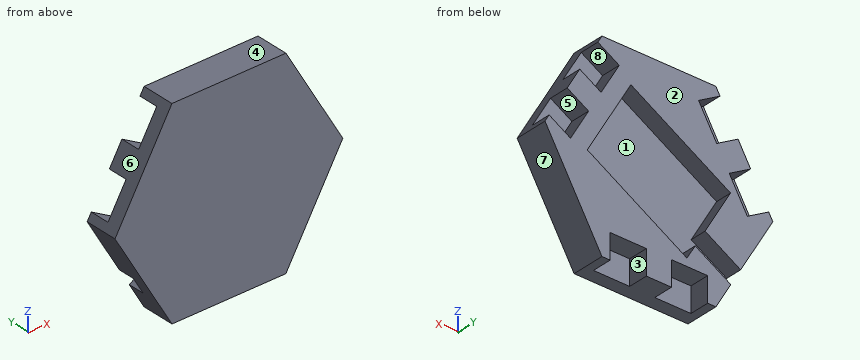
```python
from build123d import *

# Parameters (mm, degrees)
BOSS_EXTRUDE1_DEPTH     = 20
SKETCH2_W               = 22
SKETCH2_H               = 15
CUT_EXTRUDE1_DEPTH      = 12
CUT_EXTRUDE2_DEPTH      = 94.808315196
CUT_EXTRUDE2_DEPTH_BACK = 10


with BuildPart() as part:
    # Sketch1 → Boss-Extrude1 (new body)
    with BuildSketch(Plane(origin=(0, 0, 0), x_dir=(1, 0, 0), z_dir=(0, 1, 0))):
        Polygon((69.282032303, 0), (34.641016151, 60), (-34.641016151, 60), (-69.282032303, 0), (-34.641016151, -60), (34.641016151, -60), align=None)
    extrude(amount=BOSS_EXTRUDE1_DEPTH)

    # Sketch2 → Cut-Extrude1 (cut)
    with BuildSketch(Plane(origin=(0, 20, 0), x_dir=(1, 0, 0), z_dir=(0, 1, 0))):
        with Locations((-18.641016151, 52.5)):
            Rectangle(SKETCH2_W, SKETCH2_H)
        with Locations((18.641016151, 52.5)):
            Rectangle(SKETCH2_W, SKETCH2_H)
        Polygon((66.782032303, -4.330127019), (53.791651246, 3.169872981), (42.791651246, -15.882685902), (55.782032303, -23.382685902), align=None)
        Polygon((48.141016151, -36.617314098), (35.150635095, -29.117314098), (24.150635095, -48.169872981), (37.141016151, -55.669872981), align=None)
        Polygon((-37.141016151, -55.669872981), (-24.150635095, -48.169872981), (-35.150635095, -29.117314098), (-48.141016151, -36.617314098), align=None)
        Polygon((-55.782032303, -23.382685902), (-42.791651246, -15.882685902), (-53.791651246, 3.169872981), (-66.782032303, -4.330127019), align=None)
    extrude(amount=-CUT_EXTRUDE1_DEPTH, mode=Mode.SUBTRACT)

    # Sketch3 → Cut-Extrude2 (cut, two sides: drawn at the far end of the back side and taken through both)
    with BuildSketch(Plane(origin=(0, 20, 0), x_dir=(1, 0, 0), z_dir=(0, 1, 0)).offset(-CUT_EXTRUDE2_DEPTH_BACK)):
        Polygon((-43.560889132, -5.4496732), (17.060889132, -40.4496732), (43.560889132, 5.4496732), (-17.060889132, 40.4496732), align=None)
        Polygon((-22.060889132, 31.789419162), (-28.060889132, 21.397114317), (-49.711524227, 33.897114317), (-43.711524227, 44.289419162), align=None)
    extrude(amount=CUT_EXTRUDE2_DEPTH + CUT_EXTRUDE2_DEPTH_BACK, mode=Mode.SUBTRACT)


solid = part.part
```
CAD build for the part. Positions are in the model's coordinates, mm. Face numbers are marked on the shaded views. A direction names the side the tool comes from. Round coordinates to 2 decimals unless told otherwise and drop trailing zeros. Write each loop counter-clockwise with the first axis right and the second up, starting at its lowest first coordinate (ties: lowest second). Pieces come first, ordered by that corner, then holes. Notation, with made-up numbers: (44, -20.75) - (63, -20.75) arc R7 cw to (63, -15.75) - close; hole circle Ø4 at (-5.75, 27). An arc over 180 degrees is marked (long way). Write item = value, one per line. Start each with the question number.
Q1. Which spindle directions (+Z, -Z, +X, -X, +Y, -Y) get a long thin tool onto all of the face, cutting with end or side? Do the marked faces 1, 2, 3, 4 and 5. Say none if no direction does.
Q2. Band-saw the part on A-A (y = 3.5). Give the cut face in (x, z), then the cut area to 3 significant figures.
Q3. Drop flat-ended pins along their axis: pin 1 (5 mm diameter, centred on x = -4, z = 42.5, fed in from -Y); pin 2 (5 mm diameter, centred on y = 14.5, z = -31.5, fed in from +X); pin 3 (6 mm diameter, centred on y = 15, z = -55, fed in from -X); pin 4 (3.5 mm diameter, centred on y = 14.5, z = -52.5, fed in from -X). Give the stop position or say it passes through.
Q4. Band-saw the part on C-C (z = -50). Give the cut face in (x, y).
Q5. Band-saw the part on D-D (z = 43). Give the cut face in (x, y).
Q6. Probe L1, parallel to X at y = 11, z = -33; L2, parallel to Z at x = -36.5, y = 13; L3, parallel to Y at x = -1, z = 17.5. List the from-to ranges inside material, lowest first. Write a range as from..to.
Q7. Band-saw the part on B-B (x = 32). Give the cut face in (y, z), then the cut area to 3 significant figures.
Q8. Mould opens along Z. For the marked faces 6, 7 and 8 say: pulls with the +Z half, pulls with the -Z half, needs draft (parallel to the pull), parting line crosses it, or undercut.
Answers below:
q1.face_1 = +Y
q1.face_2 = +Z, -Z, +X, -X, +Y
q1.face_3 = -Z, +Y
q1.face_4 = +Z, +X, -X, +Y, -Y
q1.face_5 = +X, +Y
q2.outline = (-69.28, 0) - (-34.64, -60) - (34.64, -60) - (69.28, 0) - (34.64, 60) - (-34.64, 60) - close
q2.area = 12,500 mm2
q3.pin_1 = 0
q3.pin_2 = 52.54
q3.pin_3 = -39.26
q3.pin_4 = -39.98
q4.outline = (-40.41, 0) - (40.41, 0) - (40.41, 20) - (29.64, 20) - (29.64, 8) - (7.64, 8) - (7.64, 20) - (-7.64, 20) - (-7.64, 8) - (-29.64, 8) - (-29.64, 20) - (-40.41, 20) - close
q5.outline = (-44.46, 0) - (44.46, 0) - (44.46, 8) - (27.14, 8) - (27.14, 20) - (-27.14, 20) - (-27.14, 8) - (-44.46, 8) - close
q6.L1 = -50.23..-48.16, -24.16..-21.36, -4.16..50.23
q6.L2 = -56.78..-40.13, -26.27..-6.78, 9.53..29.9, 55.3..56.78
q6.L3 = 0..10
q7.outline = (0, -60) - (20, -60) - (20, -12.12) - (10, -12.12) - (10, 14.57) - (20, 14.57) - (20, 34.57) - (8, 34.57) - (8, 52.7) - (20, 52.7) - (20, 60) - (0, 60) - close
q7.area = 1,920 mm2
q8.face_6 = pulls with the +Z half
q8.face_7 = pulls with the -Z half
q8.face_8 = undercut
